```python
from build123d import *

# Parameters (mm, degrees)
SKETCH1_W           = 50.8
SKETCH1_H           = 50.8
SKETCH1_R           = 3.175
BOSS_EXTRUDE1_DEPTH = 3.175
SKETCH2_W           = 50.8
SKETCH2_H           = 3.175
BOSS_EXTRUDE2_DEPTH = 22.225
CUT_EXTRUDE1_REACH  = 61.653
SKETCH3_R           = 3.175


with BuildPart() as part:
    # Sketch1 → Boss-Extrude1 (new body)
    with BuildSketch(Plane(origin=(0, 0, 0), x_dir=(1, 0, 0), z_dir=(0, 1, 0))):
        Rectangle(SKETCH1_W, SKETCH1_H)
        with Locations(Location((-12.7, -12.7, 0), (0, 0, 270))):
            Circle(SKETCH1_R, mode=Mode.SUBTRACT)
        with Locations(Location((12.7, 12.7, 0), (0, 0, 90))):
            Circle(SKETCH1_R, mode=Mode.SUBTRACT)
        with Locations(Location((12.7, -12.7, 0), (0, 0, 270))):
            Circle(SKETCH1_R, mode=Mode.SUBTRACT)
        with Locations(Location((-12.7, 12.7, 0), (0, 0, 90))):
            Circle(SKETCH1_R, mode=Mode.SUBTRACT)
    extrude(amount=BOSS_EXTRUDE1_DEPTH)

    # Sketch2 → Boss-Extrude2 (add)
    with BuildSketch(Plane(origin=(0, 3.175, 0), x_dir=(1, 0, 0), z_dir=(0, 1, 0))):
        with Locations((0, 23.8125)):
            Rectangle(SKETCH2_W, SKETCH2_H)
    extrude(amount=BOSS_EXTRUDE2_DEPTH)

    # Sketch3 → Cut-Extrude1 (cut, up to next)
    with BuildSketch(Plane.XY.offset(-22.225), mode=Mode.PRIVATE) as cut_extrude1_sk1:
        with Locations((-12.7, 12.7)):
            Circle(SKETCH3_R)
    cut_extrude1_tool1 = extrude(cut_extrude1_sk1.sketch, amount=-CUT_EXTRUDE1_REACH, mode=Mode.PRIVATE) & part.part
    # Sketch3 → Cut-Extrude1 (cut, up to next)
    with BuildSketch(Plane.XY.offset(-22.225), mode=Mode.PRIVATE) as cut_extrude1_sk2:
        with Locations((12.7, 12.7)):
            Circle(SKETCH3_R)
    cut_extrude1_tool2 = extrude(cut_extrude1_sk2.sketch, amount=-CUT_EXTRUDE1_REACH, mode=Mode.PRIVATE) & part.part
    add(cut_extrude1_tool1.solids().sort_by_distance((-12.7, 12.7, -22.225))[0], mode=Mode.SUBTRACT)
    add(cut_extrude1_tool2.solids().sort_by_distance((12.7, 12.7, -22.225))[0], mode=Mode.SUBTRACT)


solid = part.part
```
Model file for the job. Use its own axes, mm. A direction names the side the tool comes from. Coordinates: 2 decimals unless noted, no trailing zeros. Loops run counter-clockwise (first coordinate to the right, second up) from the corner with the lowest first, then second, coordinate; pieces in that order, holes last. Notation, with made-up numbers: (-4, 4.25) -> (15, 4.25) arc R15 ccw to (15, 18.25) -> close; hole circle Ø11 at (50.25, 51.25). An arc over 180 degrees is marked (long way). Answer as a JSON object with one key per item and string values.
Q1. Flat gauge pins, fed straight in: P1, Ø4, axis at x = -14, y = 10, coming from the -Z side; P2, Ø1, axis at x = 1, y = 11, coming from the +Z side (3 decimals); P3, Ø10, axis at x = -12.7, z = 12.7, coming from the +Y side (3 decimals). Where does each tip first touch, or does it go through?
Report:
{"P1": "stops at z = -25.4", "P2": "stops at z = -22.225", "P3": "stops at y = 3.175"}
Q2. Cut at A-A (y = 12.7). List the corners of the cut face in (x, z) (3 decimals).
Report:
{"outline": "(-25.4, -25.4) -> (-15.875, -25.4) -> (-15.875, -22.225) -> (-25.4, -22.225) -> close; (-9.525, -25.4) -> (9.525, -25.4) -> (9.525, -22.225) -> (-9.525, -22.225) -> close; (15.875, -25.4) -> (25.4, -25.4) -> (25.4, -22.225) -> (15.875, -22.225) -> close"}
Q3. Cut at C-C (x = 12.7). List the corners of the cut face in (y, z) (3 decimals), and give its area (3 significant figures).
Report:
{"outline": "(0, -25.4) -> (9.525, -25.4) -> (9.525, -22.225) -> (3.175, -22.225) -> (3.175, -15.875) -> (0, -15.875) -> close; (0, -9.525) -> (3.175, -9.525) -> (3.175, 9.525) -> (0, 9.525) -> close; (0, 15.875) -> (3.175, 15.875) -> (3.175, 25.4) -> (0, 25.4) -> close; (15.875, -25.4) -> (25.4, -25.4) -> (25.4, -22.225) -> (15.875, -22.225) -> close", "area": "171 mm2"}
Q4. Probe probe 1 along X at (y, z) = (0.8, 12.7) (3 decimals); probe 2 along X at (y, z) = (2.5, -15); probe 3 along Y at (x, z) = (6.5, -18) (3 decimals). List the from-to ranges inside material, lowest first.
Report:
{"probe 1": "x = -25.4 to -15.875, -9.525 to 9.525, 15.875 to 25.4", "probe 2": "x = -25.4 to -14.89, -10.51 to 10.51, 14.89 to 25.4", "probe 3": "y = 0 to 3.175"}
Q5. Cut at D-D (y = 4.25). List the corners of the cut face in (x, z) (3 decimals), and give its area (3 significant figures).
Report:
{"outline": "(-25.4, -25.4) -> (25.4, -25.4) -> (25.4, -22.225) -> (-25.4, -22.225) -> close", "area": "161 mm2"}
Q6. Pull direction Z, two halves, no side cores. Call faces 3 (the flat face through (0, 3.175, 1)), 4 (the flat face through (0, 2, 25.4)), 5 (the cylindrical face through (-14.63, 1.57, 10.18)): released by +Z, released by -Z, zero draft, split by the parting line, or undercut.
Report:
{"face 3": "zero draft", "face 4": "released by +Z", "face 5": "undercut"}
Q7. 3-axis set-ups, long thin cutter, end or side, ignore diameter. For faces 1 (the flat face through (0, 14, -22.225)), 2 (the flat face through (25.4, 2, -9)): which of +Z, -Z, +X, -X, +Y, -Y reach the whole face in a straight line?
Report:
{"face 1": "+Z, +X, -X, +Y", "face 2": "+Z, -Z, +X, +Y, -Y"}
Q8. Cut at B-B (z = -12.7). List the corners of the cut face in (x, y) (3 decimals), and give its area (3 significant figures).
Report:
{"outline": "(-25.4, 0) -> (-15.875, 0) -> (-15.875, 3.175) -> (-25.4, 3.175) -> close; (-9.525, 0) -> (9.525, 0) -> (9.525, 3.175) -> (-9.525, 3.175) -> close; (15.875, 0) -> (25.4, 0) -> (25.4, 3.175) -> (15.875, 3.175) -> close", "area": "121 mm2"}
